from build123d import *

# Parameters (mm, degrees)
SKETCH014_W    = 100
SKETCH014_H    = 36.5
PAD011_DEPTH   = 6
THICKNESS002_T = 2
SKETCH015_W    = 50
SKETCH015_H    = 1
SKETCH015_W_2  = 1
SKETCH015_H_2  = 3.782178
PAD012_DEPTH   = 3
FILLET004_R    = 1.5


with BuildPart() as part:
    # Sketch014 → Pad011 (new body)
    with BuildSketch(Plane.XY):
        Rectangle(SKETCH014_W, SKETCH014_H)
    extrude(amount=PAD011_DEPTH)

    # Thickness002
    thickness002_openings = [part.faces().sort_by_distance(p)[0] for p in [
        (0, 0, 0),
    ]]
    offset(amount=THICKNESS002_T, openings=thickness002_openings)

    # Sketch015 → Pad012 (join)
    with BuildSketch(Plane.XY):
        with Locations((0, -18.75)):
            Rectangle(SKETCH015_W, SKETCH015_H)
        with Locations((50.5, 0)):
            Rectangle(SKETCH015_W_2, SKETCH015_H_2)
        with Locations((0, 18.75)):
            Rectangle(SKETCH015_W, SKETCH015_H)
        Polygon((-50, -9.125126), (-51, -9.124874), (-51, 9.125126), (-50, 9.125126), align=None)
    extrude(amount=-PAD012_DEPTH)

    # Fillet004
    fillet004_edges = [part.edges().sort_by_distance(p)[0] for p in [
        (0, 18.25, 6),
        (50, 0, 6),
        (0, -18.25, 6),
        (-50, 0, 6),
    ]]
    fillet(fillet004_edges, radius=FILLET004_R)


with BuildPart() as part_1:
    # Body004 placement: moved
    add(part.part.moved(Location((0, 0, 10))))


solid = part_1.part
Read the model definition and answer for the solid it produces. Units are mm, in the model's axes. A direction names the side the tool comes from. Round coordinates to 2 decimals unless told otherwise and drop trailing zeros. Write each loop counter-clockwise with the first axis right and the second up, starting at its lowest first coordinate (ties: lowest second). Pieces come first, ordered by that corner, then holes. Notation, with made-up numbers: (-7, 8.5) - (24, 8.5) arc R22 cw to (24, 25.5) - close; hole circle Ø9 at (48, 36.25). An arc over 180 degrees is marked (long way). Use a Markdown table: item, result.
(1) The part is cut by section D-D (y = -8). Write down the section's boundary in (x, z), then the cut area to 3 significant figures.
Reported:
| item | result |
|---|---|
| outline | (-52, 10) - (-51, 10) - (-51, 7) - (-50, 7) - (-50, 14.5) arc R1.5 cw to (-48.5, 16) - (48.5, 16) arc R1.5 cw to (50, 14.5) - (50, 10) - (52, 10) - (52, 16) arc R2 ccw to (50, 18) - (-50, 18) arc R2 ccw to (-52, 16) - close |
| area | 234 mm2 |
(2) The part is cut by section B-B (x = 43.5). Write down the section's boundary in (y, z), then the cut area to 3 significant figures.
Reported:
| item | result |
|---|---|
| outline | (-20.25, 10) - (-18.25, 10) - (-18.25, 14.5) arc R1.5 cw to (-16.75, 16) - (16.75, 16) arc R1.5 cw to (18.25, 14.5) - (18.25, 10) - (20.25, 10) - (20.25, 16) arc R2 ccw to (18.25, 18) - (-18.25, 18) arc R2 ccw to (-20.25, 16) - close |
| area | 104 mm2 |
(3) The part is cut by section C-C (z = 13.25). Write down the section's boundary in (x, y), then the cut area to 3 significant figures.
Reported:
| item | result |
|---|---|
| outline | (-52, -18.25) arc R2 ccw to (-50, -20.25) - (50, -20.25) arc R2 ccw to (52, -18.25) - (52, 18.25) arc R2 ccw to (50, 20.25) - (-50, 20.25) arc R2 ccw to (-52, 18.25) - close; hole (-50, -18.25) - (50, -18.25) - (50, 18.25) - (-50, 18.25) - close |
| area | 559 mm2 |
(4) The mould has two halves that part along X. Classify faces 4 (the flat face through (52, 0, 13)), 5 (the cylindrical face through (-51.43, 19.65, 13.04)), 6 (the flat face through (50, 0, 12)): released by +X, released by -X, zero draft, split by the parting line, or undercut.
Reported:
| item | result |
|---|---|
| face 4 | released by +X |
| face 5 | released by -X |
| face 6 | undercut |
(5) Each of these flat-tipped pins is pushed along its axis until it touches: pin 1 Ø3 at (y, z) = (11, 9.5) entering from +X; pin 2 Ø0.9 at (x, z) = (-10.5, 8) entering from +Y; pin 3 Ø0.8 at (x, z) = (50.5, 8) entering from -Y; pin 4 Ø0.8 at (y, z) = (19, 8) entering from +X. Where does it stop, or does it pass through?
Reported:
| item | result |
|---|---|
| pin 1 | x = 52 |
| pin 2 | y = 19.25 |
| pin 3 | y = -1.89 |
| pin 4 | x = 25 |
(6) The part is cut by section A-A (z = 8.5). Write down the section's boundary in (x, y), then the cut area to 3 significant figures.
Reported:
| item | result |
|---|---|
| outline | (-51, -9.12) - (-50, -9.13) - (-50, 9.13) - (-51, 9.13) - close; (-25, -19.25) - (25, -19.25) - (25, -18.25) - (-25, -18.25) - close; (-25, 18.25) - (25, 18.25) - (25, 19.25) - (-25, 19.25) - close; (50, -1.89) - (51, -1.89) - (51, 1.89) - (50, 1.89) - close |
| area | 122 mm2 |
(7) Straight lines are drawn through the part: line 1 along X through (y, z) = (-11.5, 12); line 2 along Y through (x, z) = (3, 10.25); line 3 along Z through (x, y) = (-18.5, 8.5). For each, find the intervals that lie inside material, in ascending order. Write a range as [from, to].
Reported:
| item | result |
|---|---|
| line 1 | [-52, -50], [50, 52] |
| line 2 | [-20.25, -18.25], [18.25, 20.25] |
| line 3 | [16, 18] |
(8) Which of the six approach directions +Z, -Z, +X, -X, +Y, -Y give full straight-line access (tool end or side, diameter ignored) to faces 1 (the flat face through (-1, 18.25, 12)), 2 (the flat face through (0, 19.25, 9)), 3 (the flat face through (0, -19.25, 9))?
Reported:
| item | result |
|---|---|
| face 1 | -Z |
| face 2 | -Z, +X, -X, +Y |
| face 3 | -Z, +X, -X, -Y |
